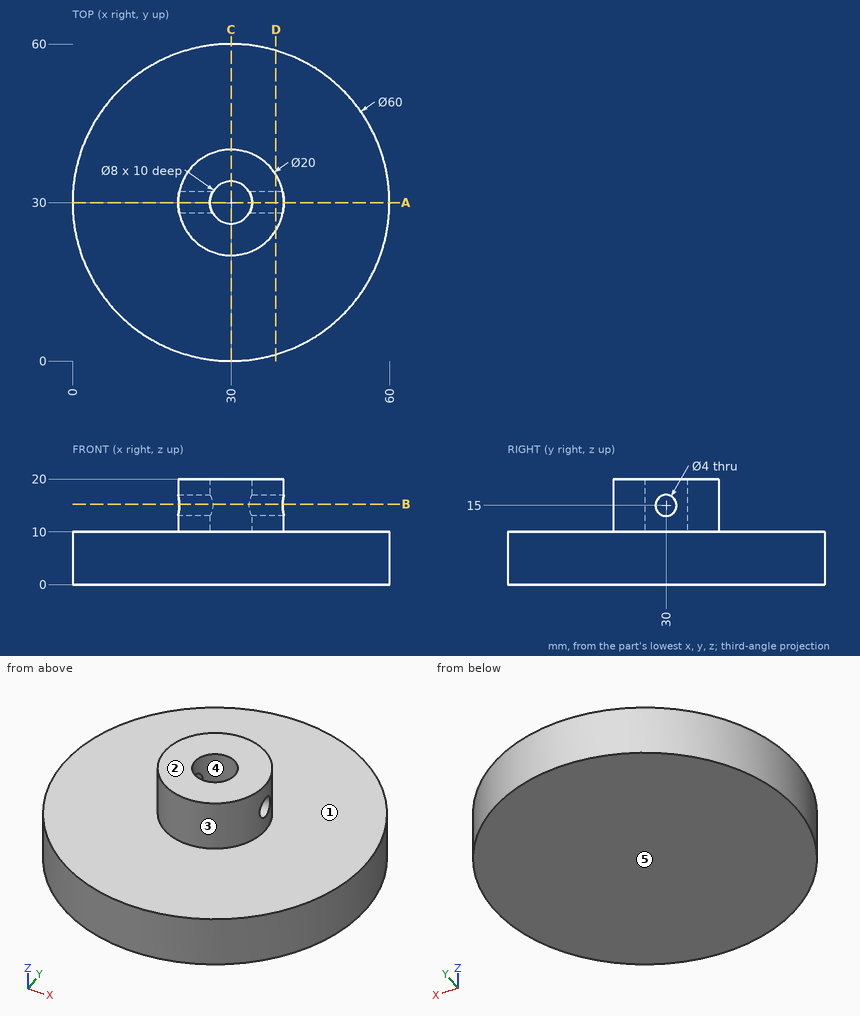
Geometry check sheet. Reference: drawing and pictorial views, mm from the part's lowest x, y, z. A direction names the side the tool comes from. Round coordinates to 2 decimals unless told otherwise and drop trailing zeros. Loops run counter-clockwise (first coordinate to the right, second up) from the corner with the lowest first, then second, coordinate; pieces in that order, holes last. Notation, with made-up numbers: M -15,39 L 31,39 A21 cw 31,46 Z; hole C -31,-23 d3. An arc over 180 degrees is marked long. Return JSON: item names as keys, results as strings. Group by question number.
(1) Section check B-B, the plane z = 15.25. Enter the section's corners in (x, y), and give its area (3 significant figures).
(2) Section check D-D, the plane x = 38.5. Enter the section's corners in (y, z), and give its area (3 significant figures).
(3) Go/stop test with flat-tipped pins: pin 1 (12 mm diameter, centred on x = 44, z = 2.5, fed in from +Y); pin 2 (4 mm diameter, centred on x = 36, z = 6, fed in from -Y); pin 3 (2.5 mm diameter, centred on x = 30, y = 30.5, fed in from +Z). Record where each tip stops, or that it passes through.
(4) Section check A-A, the plane y = 30. Enter the section's corners in (x, z).
(5) Scan lines: line 1 along X through (y, z) = (30, 12); line 2 along Z through (x, y) = (38, 30). Record each from-to range of solid material in increasing order. Write a range as [from, to].
(6) Set-up check for the marked faces 1 and 2: record each of +Z, -Z, +X, -X, +Y, -Y from which the full face is reachable in a straight line by a thin tool's end or side.
(7) Mould release check, pull along X, two halves, no side actions. Record for the marked faces 3, 4 and 5: pulls with the +X half, pulls with the -X half, needs draft (parallel to the pull), parting line crosses it, or undercut.
(8) Section check C-C, the plane x = 30. Enter the section's corners in (y, z), and give its area (3 significant figures).
Data:
{
 "1": {"outline": "M 20.2,28.02 A10 ccw 39.8,28.02 L 33.47,28.02 A4 cw 26.53,28.02 Z; M 20.2,31.98 L 26.53,31.98 A4 cw 33.47,31.98 L 39.8,31.98 A10 ccw Z", "area": "215 mm²"},
 "2": {"outline": "M 1.23,0 L 58.77,0 L 58.77,10 L 35.27,10 L 35.27,20 L 24.73,20 L 24.73,10 L 1.23,10 Z; hole C 30,15 d4", "area": "668 mm²"},
 "3": {"pin 1": "y = 58.91", "pin 2": "y = 0.27", "pin 3": "z = 10"},
 "4": {"outline": "M 0,0 L 60,0 L 60,10 L 40,10 L 40,13 L 34,13 L 34,10 L 26,10 L 26,13 L 20,13 L 20,10 L 0,10 Z; M 20,17 L 26,17 L 26,20 L 20,20 Z; M 34,17 L 40,17 L 40,20 L 34,20 Z"},
 "5": {"line 1": "[20, 26], [34, 40]", "line 2": "[0, 13], [17, 20]"},
 "6": {"face 1": "+Z", "face 2": "+Z, +X, -X, +Y, -Y"},
 "7": {"face 3": "parting line crosses it", "face 4": "undercut", "face 5": "needs draft"},
 "8": {"outline": "M 0,0 L 60,0 L 60,10 L 40,10 L 40,20 L 34,20 L 34,10 L 26,10 L 26,20 L 20,20 L 20,10 L 0,10 Z", "area": "720 mm²"}
}
